```python
from build123d import *

# Parameters (mm, degrees)
SKETCH1_W           = 9.5
SKETCH1_H           = 9.5
BOSS_EXTRUDE1_DEPTH = 5.5
SKETCH2_W           = 9.5
SKETCH2_H           = 5.5
BOSS_EXTRUDE2_DEPTH = 1.7
SKETCH3_R           = 3.5
BOSS_EXTRUDE3_DEPTH = 1
BOSS_EXTRUDE4_DEPTH = 3
SKETCH5_W           = 0.9
SKETCH5_H           = 0.6
BOSS_EXTRUDE5_DEPTH = 3.5


with BuildPart() as part:
    # Sketch1 → Boss-Extrude1 (new body)
    with BuildSketch(Plane.XY):
        Rectangle(SKETCH1_W, SKETCH1_H)
    extrude(amount=-BOSS_EXTRUDE1_DEPTH)

    # Sketch2 → Boss-Extrude2 (add)
    with BuildSketch(Plane.XZ.offset(4.75)):
        with Locations((0, -2.75)):
            Rectangle(SKETCH2_W, SKETCH2_H)
    extrude(amount=BOSS_EXTRUDE2_DEPTH)

    # Sketch3 → Boss-Extrude3 (add)
    with BuildSketch(Plane.XY):
        Circle(SKETCH3_R)
    extrude(amount=BOSS_EXTRUDE3_DEPTH)

    # Sketch4 → Boss-Extrude4 (add)
    with BuildSketch(Plane.XY.offset(1)):
        with BuildLine():
            Line((-1.60623784, 1.85), (1.60623784, 1.85))
            ThreePointArc((1.60623784, 1.85), (0, -2.45), (-1.60623784, 1.85))
        make_face()
    extrude(amount=BOSS_EXTRUDE4_DEPTH)

    # Sketch5 → Boss-Extrude5 (add)
    with BuildSketch(Plane.XZ.offset(6.45)):
        with Locations((-2.7, -3.3)):
            Rectangle(SKETCH5_W, SKETCH5_H)
        with Locations((0, -3.3)):
            Rectangle(SKETCH5_W, SKETCH5_H)
        with Locations((2.7, -3.3)):
            Rectangle(SKETCH5_W, SKETCH5_H)
    extrude(amount=BOSS_EXTRUDE5_DEPTH)


solid = part.part
```
Work out the finished part from the listing and answer in its coordinate system (mm). A direction names the side the tool comes from. Round coordinates to 2 decimals unless told otherwise and drop trailing zeros. Write each loop counter-clockwise with the first axis right and the second up, starting at its lowest first coordinate (ties: lowest second). Pieces come first, ordered by that corner, then holes. Notation, with made-up numbers: (-40, -16) -> (-14, -16) arc R30 ccw to (-14, 21) -> close; hole circle Ø11 at (1, -34). An arc over 180 degrees is marked (long way). Write each question's results on one line, items separated by ' | '.
1) Which of the six approach directions +Z, -Z, +X, -X, +Y, -Y give full straight-line access (tool end or side, diameter ignored) to faces 1 (the cylindrical face through (0.08, -2.45, 2.48)), 2 (the flat face through (-3, -8, -3.6)), 3 (the flat face through (0, -8, -3))?
Findings:
face 1: +Z | face 2: -Z, +X, -X, -Y | face 3: +Z, +X, -X, -Y
2) The part is cut by section C-C (x = 0). Write down the section's boundary in (y, z).
Findings:
outline: (-9.95, -3.6) -> (-6.45, -3.6) -> (-6.45, -5.5) -> (4.75, -5.5) -> (4.75, 0) -> (3.5, 0) -> (3.5, 1) -> (1.85, 1) -> (1.85, 4) -> (-2.45, 4) -> (-2.45, 1) -> (-3.5, 1) -> (-3.5, 0) -> (-6.45, 0) -> (-6.45, -3) -> (-9.95, -3) -> close
3) Consider line 1 along Y through (x, z) = (-2, -2.75); line 2 along Z through (x, y) = (2.75, -5.25); line 3 along Z through (x, y) = (2.5, 0.5). Determine where each line is inside the solid, lowest interval first. Write a range as [from, to].
Findings:
line 1: y = [-6.45, 4.75] | line 2: z = [-5.5, 0] | line 3: z = [-5.5, 1]
4) The part is cut by section A-A (y = -8). Write down the section's boundary in (x, z), and give its area (3 significant figures).
Findings:
outline: (-3.15, -3.6) -> (-2.25, -3.6) -> (-2.25, -3) -> (-3.15, -3) -> close; (-0.45, -3.6) -> (0.45, -3.6) -> (0.45, -3) -> (-0.45, -3) -> close; (2.25, -3.6) -> (3.15, -3.6) -> (3.15, -3) -> (2.25, -3) -> close | area: 1.62 mm²
5) The part is cut by section D-D (z = 3). Write down the section's boundary in (x, y).
Findings:
outline: (-1.61, 1.85) arc R2.45 ccw (long way) to (1.61, 1.85) -> close
6) Flat-ended cylindrical pins translate along their axes: pin 1 (0.7 mm diameter, centred on x = -2.5, y = -8.5, fed in from -Z); pin 2 (0.7 mm diameter, centred on x = 2.5, y = -9, fed in from +Z); pin 3 (1.5 mm diameter, centred on y = -7.5, z = -3, fed in from +X). Find the tip coordinate at first contact, or state that the pin passes through.
Findings:
pin 1: stops at z = -3.6 | pin 2: stops at z = -3 | pin 3: stops at x = 3.15
7) The part is cut by section B-B (y = 0). Write down the section's boundary in (x, z).
Findings:
outline: (-4.75, -5.5) -> (4.75, -5.5) -> (4.75, 0) -> (3.5, 0) -> (3.5, 1) -> (2.45, 1) -> (2.45, 4) -> (-2.45, 4) -> (-2.45, 1) -> (-3.5, 1) -> (-3.5, 0) -> (-4.75, 0) -> close
